Part model, mm, in its own coordinate system. A direction names the side the tool comes from. Round coordinates to 2 decimals unless told otherwise and drop trailing zeros. Write each loop counter-clockwise with the first axis right and the second up, starting at its lowest first coordinate (ties: lowest second). Pieces come first, ordered by that corner, then holes.
Autodesk Inventor part; units mm, degrees
ref_plane "YZ Plane" through (0, 0, 0) normal (1, 0, 0) x (0, 1, 0)
ref_plane "XZ Plane" through (0, 0, 0) normal (0, 1, 0) x (-1, 0, 0)
ref_plane "XY Plane" through (0, 0, 0) normal (0, 0, 1) x (1, 0, 0)
sketch "Sketch1" plane through (0, 0, 0) normal (0, 0, 1) x (1, 0, 0)
  circle A0 centre (0, 0) radius 4.35
  dimension "d0" = 8.7
extrude "Extrusion1" add sketch "Sketch1" along normal blind 3
sketch "Sketch2" plane through (0, 0, 0) normal (0, 0, -1) x (-1, 0, 0)
  circle A0 centre (0, 0) radius 3
  dimension "d3" = 6
extrude "Extrusion2" cut sketch "Sketch2" against normal up to next
sketch "Sketch3" plane through (0, 0, 3) normal (0, 0, 1) x (1, 0, 0)
  arc A0 (2.4721, 16.8725) -> (-2.4721, 16.8725) centre (0, 16.5) ccw
  line L0 (-4.4, 4.0792) -> (-2.4721, 16.8725)
  line L1 (4.4, 4.0792) -> (2.4721, 16.8725)
  circle A1 centre (0, 16.5) radius 0.75
  circle A2 centre (0, 13.3) radius 0.75
  circle A3 centre (0, 10.1) radius 0.75
  circle A4 centre (0, 6.9) radius 0.75
  arc A5 (-4.4, 4.0792) -> (-4.4, -4.0792) centre (0, 0) ccw
  arc A6 (4.4, -4.0792) -> (4.4, 4.0792) centre (0, 0) ccw
  arc A7 (-4.4, -4.0792) -> (4.4, -4.0792) centre (0, 0) ccw
  dimension "d8" = 8.8
  dimension "d10" = 1.5
  dimension "d13" = 1.5
  dimension "d14" = 1.5
  dimension "d15" = 1.5
extrude "Extrusion3" add sketch "Sketch3" along normal blind 2.3
sketch "Sketch4" plane through (0, 0, 5.3) normal (0, 0, 1) x (1, 0, 0)
  circle A0 centre (0, 0) radius 2.85
  circle A1 centre (0, 0) radius 4.4
  circle A2 centre (0, 0) radius 2.95
  dimension "d22" = 5.7
  dimension "d23" = 8.8
  dimension "d24" = 5.9
extrude "Extrusion4" cut sketch "Sketch4" against normal blind 1.5
sketch "Sketch5" plane through (0, 0, 3.8) normal (0, 0, 1) x (1, 0, 0)
  circle A0 centre (0, 0) radius 1.5
  dimension "d27" = 3
extrude "Extrusion5" cut sketch "Sketch5" against normal up to next
properties part number "Servomotor-1"
Q1. Cut at A-A on y = 0. Write the cut outline in (x, z).
Values follow:
outline: (-6, 3) - (-4.35, 3) - (-4.35, 0) - (-3, 0) - (-3, 3) - (-1.5, 3) - (-1.5, 3.8) - (-2.85, 3.8) - (-2.85, 5.3) - (-2.95, 5.3) - (-2.95, 3.8) - (-4.4, 3.8) - (-4.4, 5.3) - (-6, 5.3) - close; (1.5, 3) - (3, 3) - (3, 0) - (4.35, 0) - (4.35, 3) - (6, 3) - (6, 5.3) - (4.4, 5.3) - (4.4, 3.8) - (2.95, 3.8) - (2.95, 5.3) - (2.85, 5.3) - (2.85, 3.8) - (1.5, 3.8) - close
Q2. Cut at C-C on x = 0. State how many separate pieces and enclosed holes the cut face has, plus the area to 3 significant figures.
Values follow:
separate pieces: 6
enclosed holes: 0
area: 36.5 mm2
Q3. Drop flat-ended pins along their axis: pin 1 (3 mm diameter, centred on y = 2, z = 2, fed in from +X); pin 2 (2.5 mm diameter, centred on x = 0, y = 13.3, fed in from -Z); pin 3 (1 mm diameter, centred on y = 13, z = 4, fed in from -X). Give the stop position or say it passes through.
Values follow:
pin 1: stops at x = 5.93
pin 2: stops at z = 3
pin 3: stops at x = -3.13
Q4. Wall check: L1, parallel to Y at x = 0, z = 3.2; L2, parallel to Z at x = -2.5, y = 7.5; L3, parallel to Z at x = 0.5, y = -3.5. Give the ranges that are in metal, low to high.
Values follow:
L1: y = -6 to -1.5, 1.5 to 6.15, 7.65 to 9.35, 10.85 to 12.55, 14.05 to 15.75, 17.25 to 19
L2: z = 3 to 5.3
L3: z = 0 to 3.8
Q5. Mould opens along Y. For faces 4 (the cylindrical face through (0, -6, 4)), 5 (the cylindrical face through (0, 19, 4)), 6 (the cylindrical face through (-0.163, 10.832, 4.134)) say: +Y half, -Y half, draft (parallel to the pull), parting line (faces both ways), or undercut.
Values follow:
face 4: parting line
face 5: +Y half
face 6: undercut
Q6. Which spindle directions (+Z, -Z, +X, -X, +Y, -Y) get a long thin tool onto all of the face, cutting with end or side? Do faces 1 (the cylindrical face through (3, 0, 1)), 2 (the flat face through (1, 7, 5.3)), 3 (the cylindrical face through (4.197, 1.322, 4.56)). Say none if no direction does.
Values follow:
face 1: -Z
face 2: +Z, +X, -X, +Y, -Y
face 3: +Z
Q7. Cut at B-B on z = 4.15. Write the cut outline in (x, y).
Values follow:
outline: (-4.4, 4.08) arc R6 ccw (long way) to (4.4, 4.08) - (2.47, 16.87) arc R2.5 ccw to (-2.47, 16.87) - close; circle Ø5.9 at (0, 0); hole circle Ø8.8 at (0, 0); hole circle Ø5.7 at (0, 0); hole circle Ø1.5 at (0, 6.9); hole circle Ø1.5 at (0, 10.1); hole circle Ø1.5 at (0, 13.3); hole circle Ø1.5 at (0, 16.5)
Q8. Cut at D-D on z = 0.4. Write the cut outline in (x, y).
Values follow:
outline: circle Ø8.7 at (0, 0); hole circle Ø6 at (0, 0)
